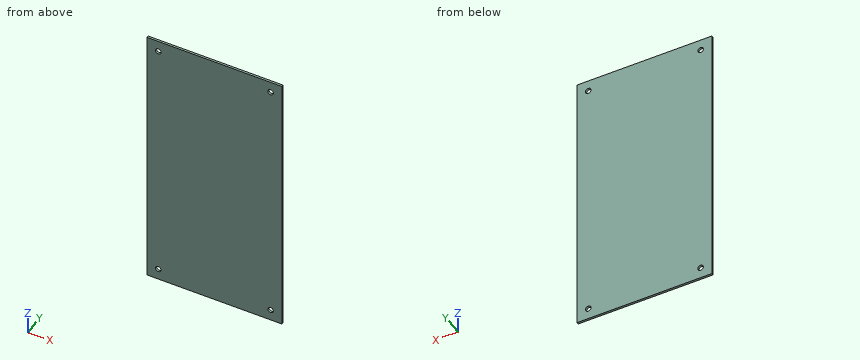
```python
from build123d import *

# Parameters (mm, degrees)
F0_W     = 304.8
F0_H     = 609.6
F2_DEPTH = 4.7625
F1_D     = 12.7


with BuildPart() as f2:
    # F0 (on Front) → F2 (new body)
    with BuildSketch(Plane.XZ):
        Rectangle(F0_W, F0_H)
    extrude(amount=F2_DEPTH)

    # F1 (through all)
    with Locations(Plane(origin=(0, 0, 0), x_dir=(1, 0, 0), z_dir=(0, 1, 0))):
        with Locations((-127, 279.4), (127, 279.4), (-127, -279.4), (127, -279.4)):
            Hole(F1_D / 2)


solid = f2.part
```
Geometry check sheet. Reference: the model listing, model coordinates, mm. Give positions to 0.01 mm unless a question says otherwise; leave off trailing zeros. Order: outer loops, then holes, each group sorted by start corner. A loop starts at its lowest first (then second) coordinate and runs counter-clockwise, first axis right, second up.
1. Section check A-A, the plane x = -127. Enter the section's corners in (y, z).
2. Gauge pin test, flat end, axial feed: pin 1 Ø20.5 at (x, z) = (-127, -279.4) entering from -Y. Record the tip position at first contact, or that the pin passes through.
3. Thickness scan on L1, parallel to Z at x = -127, y = -1.9; L2, parallel to X at y = -2.25, z = 279.4; L3, parallel to X at y = -1.7, z = 275. Record the ranges inside material, lowest first.
4. Section check B-B, the plane z = -279.4. Enter the section's corners in (x, y).
Values follow:
1. outline: (-4.76, -304.8) - (0, -304.8) - (0, -285.75) - (-4.76, -285.75) - close; (-4.76, -273.05) - (0, -273.05) - (0, 273.05) - (-4.76, 273.05) - close; (-4.76, 285.75) - (0, 285.75) - (0, 304.8) - (-4.76, 304.8) - close
2. pin 1: stops at y = -4.76
3. L1: z = -304.8 to -285.75, -273.05 to 273.05, 285.75 to 304.8
3. L2: x = -152.4 to -133.35, -120.65 to 120.65, 133.35 to 152.4
3. L3: x = -152.4 to -131.58, -122.42 to 122.42, 131.58 to 152.4
4. outline: (-152.4, -4.76) - (-133.35, -4.76) - (-133.35, 0) - (-152.4, 0) - close; (-120.65, -4.76) - (120.65, -4.76) - (120.65, 0) - (-120.65, 0) - close; (133.35, -4.76) - (152.4, -4.76) - (152.4, 0) - (133.35, 0) - close
